Geometry check sheet. Reference: the model listing, model coordinates, mm. A direction names the side the tool comes from. Round coordinates to 2 decimals unless told otherwise and drop trailing zeros. Loops run counter-clockwise (first coordinate to the right, second up) from the corner with the lowest first, then second, coordinate; pieces in that order, holes last. Notation, with made-up numbers: (-20, 84) - (38, 84) arc R17 cw to (38, 111) - close; hole circle Ø5 at (64.25, -34.5). An arc over 180 degrees is marked (long way). Answer in a Markdown table with one row per item. Add a question column.
```python
from build123d import *

# Parameters (mm, degrees)
EXTRUDE_1_DEPTH     = 250
SKETCH_2_R          = 4.1
CUT_EXTRUDE_1_DEPTH = 10


with BuildPart() as part:
    # Эскиз1 → Вытянуть-Тонкостенный1 (new body)
    with BuildSketch(Plane(origin=(0, 0, 0), x_dir=(0, 0, -1), z_dir=(1, 0, 0))):
        Polygon((40, 0), (0, 0), (0, 40), (3, 40), (3, 3), (40, 3), align=None)
    extrude(amount=EXTRUDE_1_DEPTH)

    # Эскиз2 → Вырез-Вытянуть1 (cut)
    with BuildSketch(Plane.XY):
        with Locations((35, 20)):
            Circle(SKETCH_2_R)
        with Locations((85, 20)):
            Circle(SKETCH_2_R)
        with Locations((135, 20)):
            Circle(SKETCH_2_R)
        with Locations((185, 20)):
            Circle(SKETCH_2_R)
    extrude(amount=-CUT_EXTRUDE_1_DEPTH, mode=Mode.SUBTRACT)


solid = part.part
```
Q1. Set-up check for faces 4 (the flat face through (123, 3, -21)), 5 (the cylindrical face through (81.746, 17.505, -1.479)): record each of +Z, -Z, +X, -X, +Y, -Y from which the full face is reachable in a straight line by a thin tool's end or side.
Q2. Cross-section at C-C, the plane x = 198. Enter the section's corners in (y, z).
Q3. Depth check by flat-ended pin: P1, Ø8, axis at x = 144, y = 17, coming from the -Z side; P2, Ø11, axis at x = 139, z = -26, coming from the +Y side. Enter the tip coordinate at first touch or a pass-through.
Q4. Scan lines: line 1 (Y direction, x = 85, z = -1.8); line 2 (Z direction, x = 157.5, y = 17.5); line 3 (Y direction, x = 97, z = -27). Record each from-to range of solid material in increasing order. Write a range as from..to.
Q5. Cross-section at B-B, the plane y = 20. Enter the section's corners in (x, z).
Q6. Cross-section at A-A, the plane x = 135. Enter the section's corners in (y, z), plus the area to 3 significant figures.
Q7. Cross-section at D-D, the plane z = -12. Enter the section's corners in (x, y), plus the area to 3 significant figures.
Q8. Release check for a two-part mould opening along Y. For faces 1 (the flat face through (123, 0, -20)), 2 (the cylindrical face through (31.746, 17.505, -1.479)), 3 (the flat face through (0, 2, -11)) record: +Y half, -Y half, draft (parallel to the pull), parting line (faces both ways), or undercut.
Check sheet entries:
| question | item | result |
|---|---|---|
| 1 | face 4 | -Z, +X, -X, +Y |
| 1 | face 5 | +Z, -Z |
| 2 | outline | (0, -40) - (3, -40) - (3, -3) - (40, -3) - (40, 0) - (0, 0) - close |
| 3 | P1 | z = -3 |
| 3 | P2 | y = 3 |
| 4 | line 1 | 0..15.9, 24.1..40 |
| 4 | line 2 | -3..0 |
| 4 | line 3 | 0..3 |
| 5 | outline | (0, -3) - (30.9, -3) - (30.9, 0) - (0, 0) - close; (39.1, -3) - (80.9, -3) - (80.9, 0) - (39.1, 0) - close; (89.1, -3) - (130.9, -3) - (130.9, 0) - (89.1, 0) - close; (139.1, -3) - (180.9, -3) - (180.9, 0) - (139.1, 0) - close; (189.1, -3) - (250, -3) - (250, 0) - (189.1, 0) - close |
| 6 | outline | (0, -40) - (3, -40) - (3, -3) - (15.9, -3) - (15.9, 0) - (0, 0) - close; (24.1, -3) - (40, -3) - (40, 0) - (24.1, 0) - close |
| 6 | area | 206 mm² |
| 7 | outline | (0, 0) - (250, 0) - (250, 3) - (0, 3) - close |
| 7 | area | 750 mm² |
| 8 | face 1 | -Y half |
| 8 | face 2 | undercut |
| 8 | face 3 | draft |
